Here's the drawing with two shaded views (mm, measured from the low corner). I have some questions. A direction names the side the tool comes from. Give positions to 0.01 mm unless a question says otherwise; leave off trailing zeros. Order: outer loops, then holes, each group sorted by start corner. A loop starts at its lowest first (then second) coordinate and runs counter-clockwise, first axis right, second up. Notation, with made-up numbers: M -10.5,26.25 L -4.5,26.25 A22 cw -4.5,58.25 Z; hole C 15.5,11 d6. An arc over 180 degrees is marked long. One line per question, with ' | ' between items. Start each with the question number.
1) I'm going to push flat-ended pins straight in: pin 1 Ø8 at (x, z) = (14, 8.5) entering from -Y; pin 2 Ø6 at (y, z) = (15.5, 3.5) entering from +X; pin 3 Ø4 at (x, z) = (12.5, 4.5) entering from +Y. Where does each tip first touch, or does it pass through?
2) If we section it at D-D, the plane z = 4: Please give me the cut outline in (x, y).
3) If we section it at A-A, the plane x = 8.89: Please give me the cut outline in (y, z), plus the area to 3 significant figures.
4) If we section it at C-C, the plane z = 2: Please give me the cut outline in (x, y), plus the area to 3 significant figures.
5) Thinking about a two-plate mould opening in X: for the marked faces 4, 5 and 6, which applies, +X half, -X half, draft (parallel to the pull), parting line (faces both ways), or undercut?
6) Please list where these lines run through material, in increasing order: line 1 along Y through (x, z) = (8.89, 0.9); line 2 along Y through (x, z) = (8.89, 2.5). Write a range as [from, to].
7) For the marked faces 1, 2 and 3, which set-ups out of +Z, -Z, +X, -X, +Y, -Y let a thin tool reach every point of the face, with its end or its side?
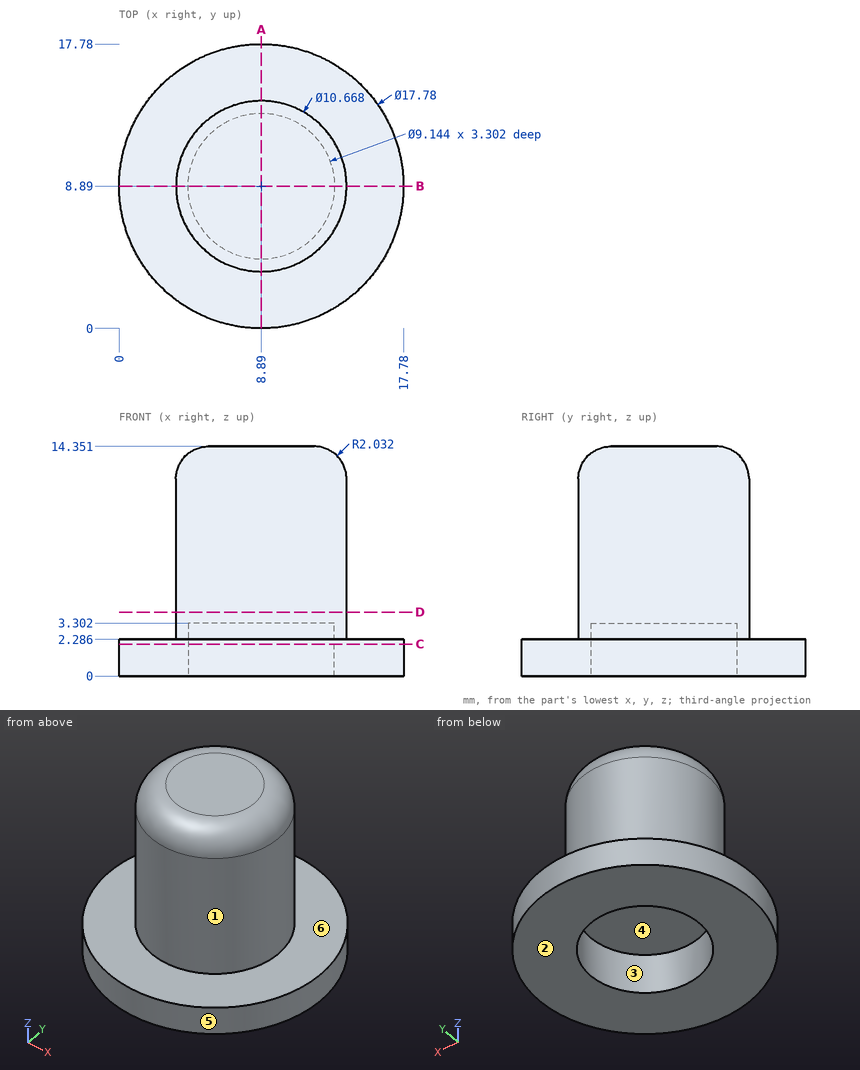
Results found:
1) pin 1: stops at y = 3.67 | pin 2: stops at x = 16.9 | pin 3: stops at y = 13.98
2) outline: C 8.89,8.89 d10.67
3) outline: M 0,0 L 4.32,0 L 4.32,3.3 L 13.46,3.3 L 13.46,0 L 17.78,0 L 17.78,2.29 L 14.22,2.29 L 14.22,12.32 A2.03 ccw 12.19,14.35 L 5.59,14.35 A2.03 ccw 3.56,12.32 L 3.56,2.29 L 0,2.29 Z | area: 137 mm²
4) outline: C 8.89,8.89 d17.78; hole C 8.89,8.89 d9.14 | area: 183 mm²
5) face 4: undercut | face 5: parting line | face 6: draft
6) line 1: y = [0, 4.32], [13.46, 17.78] | line 2: y = [3.56, 4.32], [13.46, 14.22]
7) face 1: +Z | face 2: -Z, +X, -X, +Y, -Y | face 3: -Z
